Geometry check sheet. Reference: the model listing, model coordinates, mm. Face numbers are marked on the shaded views. A direction names the side the tool comes from. Give positions to 0.01 mm unless a question says otherwise; leave off trailing zeros. Write each loop counter-clockwise with the first axis right and the second up, starting at its lowest first coordinate (ties: lowest second). Pieces come first, ordered by that corner, then holes. Notation, with made-up numbers: M -25.5,55.25 L -20.5,55.25 A33 cw -20.5,89.25 Z; hole C 2,39.25 d9. An arc over 180 degrees is marked long. Write each question's results on one line, items separated by ' | '.
```python
from build123d import *

# Parameters (mm, degrees)
SKETCH_R           = 14.5
PAD_DEPTH          = 2
SKETCH001_R        = 8
PAD001_DEPTH       = 9.9
POCKET_DEPTH       = 5
PAD002_DEPTH       = 3
POLARPATTERN_COUNT = 4
SKETCH004_R        = 6
POCKET001_DEPTH    = 2.9
FILLET_R           = 1
FILLET001_R        = 1
FILLET002_R        = 1


with BuildPart() as part:
    # Sketch → Pad (new body)
    with BuildSketch(Plane.XY):
        Circle(SKETCH_R)
    extrude(amount=PAD_DEPTH)

    # Sketch001 (on Face3 of Pad) → Pad001 (join)
    with BuildSketch(Plane.XY.offset(2)):
        Circle(SKETCH001_R)
    extrude(amount=PAD001_DEPTH)

    # Sketch002 (on Face5 of Pad001) → Pocket (cut)
    with BuildSketch(Plane.XY.offset(11.9)):
        Polygon((3.626666, -3.390946), (4.749979, 1.445312), (1.123312, 4.836258), (-3.626666, 3.390946), (-4.749979, -1.445312), (-1.123312, -4.836258), align=None)
    extrude(amount=-POCKET_DEPTH, mode=Mode.SUBTRACT)

    # Sketch003 (on Face2 of Pocket) → Pad002 (join)
    with BuildSketch(Plane(origin=(0, 0, 0), x_dir=(1, 0, 0), z_dir=(0, 0, -1))):
        with BuildLine():
            ThreePointArc((11, 3.5), (7.5, 0), (11, -3.5))
            Line((14.5, -3.5), (11, -3.5))
            Line((14.5, 3.5), (14.5, -3.5))
            Line((11, 3.5), (14.5, 3.5))
        make_face()
    pad002 = extrude(amount=PAD002_DEPTH)

    # PolarPattern: Pad002 ×4 about axis
    polarpattern_axis = Axis((0, 0, 0), (0, 0, -1))
    for i in range(1, POLARPATTERN_COUNT):
        add(pad002.rotate(polarpattern_axis, i * 360 / POLARPATTERN_COUNT))

    # Sketch004 (on Face4 of PolarPattern) → Pocket001 (cut)
    with BuildSketch(Plane(origin=(0, 0, 0), x_dir=(1, 0, 0), z_dir=(0, 0, -1))):
        Circle(SKETCH004_R)
    extrude(amount=-POCKET001_DEPTH, mode=Mode.SUBTRACT)

    # Fillet
    fillet_edges = [part.edges().sort_by_distance(p)[0] for p in [
        (-8, 0, 2),
    ]]
    fillet(fillet_edges, radius=FILLET_R)

    # Fillet001
    fillet001_edges = [part.edges().sort_by_distance(p)[0] for p in [
        (-8, 0, 11.9),
    ]]
    fillet(fillet001_edges, radius=FILLET001_R)

    # Fillet002
    fillet002_edges = [part.edges().sort_by_distance(p)[0] for p in [
        (4.188323, -0.972817, 11.9),
        (1.251677, -4.113602, 11.9),
        (-2.936646, -3.140785, 11.9),
        (-4.188323, 0.972817, 11.9),
        (-1.251677, 4.113602, 11.9),
        (2.936646, 3.140785, 11.9),
    ]]
    fillet(fillet002_edges, radius=FILLET002_R)


solid = part.part
```
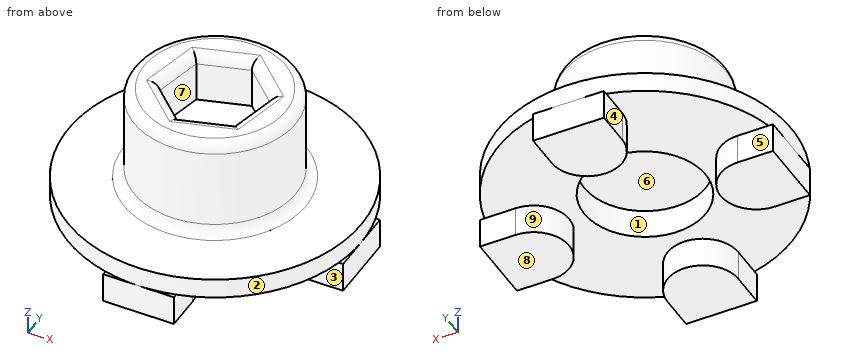
Q1. Depth check by flat-ended pin: P1, Ø0.5, axis at x = 1.5, y = 14.5, coming from the +Z side; P2, Ø7, axis at x = 0, y = 0, coming from the +Z side; P3, Ø2.5, axis at x = -13.5, z = -1.5, coming from the +Y side; P4, Ø2, axis at x = -1, z = 2, coming from the -Y side. Enter the tip coordinate at first touch or a pass-through.
Answer key:
P1: stops at z = 2 | P2: stops at z = 6.9 | P3: stops at y = 3.5 | P4: stops at y = -14.5
Q2. Material ranges on probe 1 along Y at (x, z) = (0, 1.35); probe 2 along Z at (x, y) = (-8.5, -6); probe 3 along Z at (x, y) = (2.75, -1.75), recorded low to high. Write a range as [from, to].
Answer key:
probe 1: y = [-14.5, -6], [6, 14.5] | probe 2: z = [0, 2] | probe 3: z = [2.9, 6.9]
Q3. Section check A-A (z = 7.75). Enter the section's corners in (x, y).
Answer key:
outline: C 0,0 d16; hole M -4.75,-1.45 L -1.12,-4.84 L 3.63,-3.39 L 4.75,1.45 L 1.12,4.84 L -3.63,3.39 Z
Q4. Section check B-B (x = 9.75). Enter the section's corners in (y, z), then the cut area to 3 significant figures.
Answer key:
outline: M -10.73,0 L -3.27,0 L -3.27,-3 L 3.27,-3 L 3.27,0 L 10.73,0 L 10.73,2 L -10.73,2 Z | area: 62.5 mm2
Q5. Section check C-C (z = 5). Enter the section's corners in (x, y).
Answer key:
outline: C 0,0 d16
Q6. Release check for a two-part mould opening along Y. For the marked faces 6, 7, 8 and 9 record: released by +Y, released by -Y, zero draft, split by the parting line, or undercut.
Answer key:
face 6: undercut | face 7: undercut | face 8: zero draft | face 9: split by the parting line
Q7. Access from +Z, -Z, +X, -X, +Y, -Y to the whole of each face (thin tool, end or side, straight path). Record for the marked faces 1, 2, 3, 4 and 5.
Answer key:
face 1: -Z | face 2: +Z | face 3: -Z, +X, -X, -Y | face 4: -Z, -X, +Y, -Y | face 5: -Z, +X, -X, +Y
